from build123d import *

# Parameters (mm, degrees)
SKETCH3_W           = 136.24
SKETCH3_H           = 150.17
BOSS_EXTRUDE1_DEPTH = 30
CUT_EXTRUDE1_DEPTH  = 30
BOSS_EXTRUDE2_DEPTH = 10


with BuildPart() as part:
    # Sketch3 → Boss-Extrude1 (new body)
    with BuildSketch(Plane(origin=(0, 0, 0), x_dir=(0, 0, -1), z_dir=(1, 0, 0))):
        Rectangle(SKETCH3_W, SKETCH3_H)
    extrude(amount=BOSS_EXTRUDE1_DEPTH)

    # Sketch4 → Cut-Extrude1 (cut)
    with BuildSketch(Plane.ZY):
        Polygon((-68.12, 75.085), (-48.12, 75.085), (-68.12, 55.085), align=None)
        Polygon((68.12, 75.085), (68.12, 55.085), (48.12, 75.085), align=None)
        Polygon((-68.12, -75.085), (-68.12, -55.085), (-48.12, -75.085), align=None)
        Polygon((68.12, -75.085), (68.12, -55.085), (48.12, -75.085), align=None)
        Polygon((25.49577004, -20), (29.49577004, -20), (29.49577004, -40), (25.49577004, -40), (-4.50422996, -40), (-4.50422996, -20), align=None)
    extrude(amount=-CUT_EXTRUDE1_DEPTH, mode=Mode.SUBTRACT)

    # Sketch6 → Boss-Extrude2 (add)
    with BuildSketch(Plane(origin=(30, 0, 0), x_dir=(0, 0, -1), z_dir=(1, 0, 0))):
        Polygon((-68.12, 55.085), (-48.12, 75.085), (48.12, 75.085), (68.12, 55.085), (68.12, -55.085), (48.12, -75.085), (-48.12, -75.085), (-68.12, -55.085), align=None)
    extrude(amount=BOSS_EXTRUDE2_DEPTH)


solid = part.part
Verification items for the finished model (mm, model axes). A direction names the side the tool comes from. Give positions to 0.01 mm unless a question says otherwise; leave off trailing zeros. Write each loop counter-clockwise with the first axis right and the second up, starting at its lowest first coordinate (ties: lowest second). Pieces come first, ordered by that corner, then holes. Notation, with made-up numbers: M 84.25,44.25 L 101.25,44.25 A12 ccw 101.25,59.25 Z; hole C -22.5,-36 d1. An arc over 180 degrees is marked long. Put each result on its own line as item: value. Start each with the question number.
1. Section check A-A (x = 16.5). Record the cut outline in (y, z) (3 decimals).
2. Set-up check for faces 4 (the face through (15, -20, 13)), 5 (the face through (19.72, 65.225, -57.98)): record each of +Z, -Z, +X, -X, +Y, -Y from which the full face is reachable in a straight line by a thin tool's end or side.
3. Go/stop test with flat-tipped pins: pin 1 Ø16 at (y, z) = (-31.5, 9.5) entering from -X; pin 2 Ø6 at (x, y) = (5.5, 59) entering from +Z (3 decimals); pin 3 Ø8 at (y, z) = (28.5, 8) entering from -X. Record where each tip stops, or that it passes through.
4. Scan lines: line 1 along Y through (x, z) = (24, 13.5) (3 decimals); line 2 along Z through (x, y) = (19, -21); line 3 along Y through (x, z) = (11.5, 61) (3 decimals). Record each from-to range of solid material in increasing order. Write a range as [from, to].
5. Section check D-D (z = 54.5). Record the cut outline in (x, y) (3 decimals).
6. Section check C-C (z = -1). Record the cut outline in (x, y) (3 decimals).
7. Draft check along Z on faces 1 (the face through (40, 1, -1)), 2 (the face through (19.72, -65.225, 57.98)), 3 (the face through (15, -40, 12)). Enter one of: +Z half, -Z half, draft (parallel to the pull), parting line (faces both ways), or undercut.
8. Section check B-B (x = 36.5). Record the cut outline in (y, z) (3 decimals).
Answer list:
1. outline: M -75.085,-48.12 L -55.085,-68.12 L 55.085,-68.12 L 75.085,-48.12 L 75.085,48.12 L 55.085,68.12 L -55.085,68.12 L -75.085,48.12 Z; hole M -40,-4.504 L -20,-4.504 L -20,29.496 L -40,29.496 Z
2. face 4: -X
2. face 5: -Z, +X, -X, +Y
3. pin 1: x = 30
3. pin 2: z = 67.205
3. pin 3: x = 0
4. line 1: [-75.085, -40], [-20, 75.085]
4. line 2: [-68.12, -4.5], [29.5, 68.12]
4. line 3: [-62.205, 62.205]
5. outline: M 0,-68.705 L 40,-68.705 L 40,68.705 L 0,68.705 Z
6. outline: M 0,-75.085 L 40,-75.085 L 40,75.085 L 0,75.085 L 0,-20 L 30,-20 L 30,-40 L 0,-40 Z
7. face 1: draft
7. face 2: +Z half
7. face 3: undercut
8. outline: M -75.085,-48.12 L -55.085,-68.12 L 55.085,-68.12 L 75.085,-48.12 L 75.085,48.12 L 55.085,68.12 L -55.085,68.12 L -75.085,48.12 Z
